```python
from build123d import *

# Parameters (mm, degrees)
SKETCH1_W               = 12.409227922
SKETCH1_H               = 27.718567262
SKETCH1_R               = 1
SKETCH1_W_2             = 8
SKETCH1_H_2             = 18.5
BOSS_EXTRUDE1_DEPTH     = 10
SKETCH6_W               = 12.409227922
SKETCH6_H               = 4.603346058
BOSS_EXTRUDE3_DEPTH     = 15
SKETCH7_R               = 3.1
CUT_EXTRUDE4_DEPTH      = 2.25
SKETCH8_W               = 11.323212184
SKETCH8_H               = 4
CUT_EXTRUDE5_DEPTH      = 1.25
CUT_EXTRUDE7_DEPTH      = 31.392767012
CUT_EXTRUDE7_DEPTH_BACK = 31.392767012
SKETCH9_R               = 1.5
SKETCH9_R_2             = 0.5
FILLET2_R               = 5
SKETCH10_R              = 3.380365375
CUT_EXTRUDE8_DEPTH      = 0.5
CHAMFER3_SIZE           = 2
FILLET3_R               = 5


with BuildPart() as part:
    # Sketch1 → Boss-Extrude1 (new body)
    with BuildSketch(Plane(origin=(0, 0, 0), x_dir=(0, 0, -1), z_dir=(1, 0, 0))):
        with Locations((1.233520205, 9.89974551)):
            Rectangle(SKETCH1_W, SKETCH1_H)
        with Locations((1.233520205, 20.798227972)):
            Circle(SKETCH1_R, mode=Mode.SUBTRACT)
        with Locations((1.233520205, -1.111772028)):
            Circle(SKETCH1_R, mode=Mode.SUBTRACT)
        with Locations((1.233520205, 9.843227972)):
            Rectangle(SKETCH1_W_2, SKETCH1_H_2, mode=Mode.SUBTRACT)
    extrude(amount=BOSS_EXTRUDE1_DEPTH)

    # Sketch6 → Boss-Extrude3 (add)
    with BuildSketch(Plane.ZY):
        with Locations((-1.233520205, 21.457356112)):
            Rectangle(SKETCH6_W, SKETCH6_H)
    extrude(amount=BOSS_EXTRUDE3_DEPTH)

    # Sketch7 → Cut-Extrude4 (cut)
    with BuildSketch(Plane.XZ.offset(-19.155683083)):
        with Locations(Location((-9.660045294, -1.233520205, 0), (0, 0, 270))):
            Circle(SKETCH7_R)
    extrude(amount=-CUT_EXTRUDE4_DEPTH, mode=Mode.SUBTRACT)

    # Sketch8 → Cut-Extrude5 (cut)
    with BuildSketch(Plane.XZ.offset(-19.155683083)):
        with Locations((-5.661606092, -1.303442539)):
            Rectangle(SKETCH8_W, SKETCH8_H)
    extrude(amount=-CUT_EXTRUDE5_DEPTH, mode=Mode.SUBTRACT)

    # Sketch9 → Cut-Extrude7 (cut, two sides: drawn at the far end of the back side and taken through both)
    with BuildSketch(Plane.XZ.offset(-21.405683083).offset(-CUT_EXTRUDE7_DEPTH_BACK)):
        with Locations(Location((-9.660045294, -1.233520205, 0), (0, 0, 270))):
            Circle(SKETCH9_R)
        with Locations(Location((-1.660045294, -1.233520205, 0), (0, 0, 270))):
            Circle(SKETCH9_R_2)
    extrude(amount=CUT_EXTRUDE7_DEPTH + CUT_EXTRUDE7_DEPTH_BACK, mode=Mode.SUBTRACT)

    # Fillet2
    fillet2_edges = [part.edges().sort_by_distance(p)[0] for p in [
        (-15, 21.457356112, -7.438134166),
        (-15, 21.457356112, 4.971093756),
    ]]
    fillet(fillet2_edges, radius=FILLET2_R)

    # Sketch10 → Cut-Extrude8 (cut)
    with BuildSketch(Plane(origin=(0, 23.759029141, 0), x_dir=(1, 0, 0), z_dir=(0, 1, 0))):
        with Locations(Location((-9.660045294, 1.233520205, 0), (0, 0, 270))):
            Circle(SKETCH10_R)
    extrude(amount=-CUT_EXTRUDE8_DEPTH, mode=Mode.SUBTRACT)

    # Chamfer3
    # the kernel refuses this chamfer: 2 mm, written as the material it takes off along each edge
    with BuildSketch(Plane(origin=(-5.143365976, -3.959538121, -7.438134166), x_dir=(0, 0.9996219169112968, -0.027495876610586487), z_dir=(1, 0, 0))) as chamfer3_piece_1:
        Polygon((CHAMFER3_SIZE * 0.999621916911, CHAMFER3_SIZE * 0.0274958766106), (-CHAMFER3_SIZE * 0.0274958766106, CHAMFER3_SIZE * 0.999621916911), (0, 0), align=None)
    extrude(amount=20.286731952, mode=Mode.SUBTRACT)
    with BuildSketch(Plane(origin=(-5.143365976, -3.959538121, 4.971093756), x_dir=(0, 0.9996219169112968, 0.027495876610586487), z_dir=(1, 0, 0))) as chamfer3_piece_2:
        Polygon((CHAMFER3_SIZE * 0.999621916911, -CHAMFER3_SIZE * 0.0274958766106), (-CHAMFER3_SIZE * 0.0274958766106, -CHAMFER3_SIZE * 0.999621916911), (0, 0), align=None)
    extrude(amount=20.286731952, mode=Mode.SUBTRACT)
    with BuildSketch(Plane(origin=(-10, 23.759029141, 4.971093756), x_dir=(0, 0.02749587661058563, -0.9996219169112968), z_dir=(1, 0, 0)), Plane(origin=(15.143365976, 23.759029141, -7.438134166), x_dir=(0, 0.027495876610585623, 0.9996219169112968), z_dir=(-1, 0, 0))) as chamfer3_piece_3:
        Polygon((CHAMFER3_SIZE * 0.999621916911, -CHAMFER3_SIZE * 0.0274958766106), (-CHAMFER3_SIZE * 0.0274958766106, -CHAMFER3_SIZE * 0.999621916911), (0, 0), align=None)
    extrude(amount=25.143365976, mode=Mode.SUBTRACT)
    with BuildSketch(Plane(origin=(-15, 23.759029141, -2.438134166), x_dir=(0.9996219169112968, 0.027495876610585623, 0), z_dir=(0, 0, 1))) as chamfer3_piece_4:
        Polygon((CHAMFER3_SIZE * 0.999621916911, -CHAMFER3_SIZE * 0.0274958766106), (-CHAMFER3_SIZE * 0.0274958766106, -CHAMFER3_SIZE * 0.999621916911), (0, 0), align=None)
    extrude(amount=2.409227923, mode=Mode.SUBTRACT)
    with BuildSketch(Plane(origin=(-10, 23.759029141, -0.028906244), x_dir=(-1, 0, 0), z_dir=(0, 0, -1))) as chamfer3_piece_5:
        Polygon((5 - CHAMFER3_SIZE, 0), (5, -CHAMFER3_SIZE), (5, 0), align=None)
    revolve(axis=Axis((-10, 23.759029141, -0.028906244), (0, 1, 0)), revolution_arc=90, mode=Mode.SUBTRACT)
    with BuildSketch(Plane(origin=(-10, 23.759029141, -2.438134166), x_dir=(-1, 0, 0), z_dir=(0, 0, 1))) as chamfer3_piece_6:
        Polygon((5 - CHAMFER3_SIZE, 0), (5, CHAMFER3_SIZE), (5, 0), align=None)
    revolve(axis=Axis((-10, 23.759029141, -2.438134166), (0, -1, 0)), revolution_arc=90, mode=Mode.SUBTRACT)

    # Fillet3
    # the kernel refuses this fillet: 5 mm, written as the material it adds along each edge
    with BuildSketch(Plane(origin=(0, 19.155683083, 9.196557461), x_dir=(-1, 0, 0), z_dir=(0, 0, -1))) as fillet3_piece_1_section:
        with BuildLine():
            CenterArc((FILLET3_R, -FILLET3_R), FILLET3_R, 90, 90)
            Line((0, -FILLET3_R), (0, 0))
            Line((0, 0), (FILLET3_R, 0))
        make_face()
    fillet3_piece_1 = extrude(amount=29.134691627, mode=Mode.PRIVATE)
    fillet3_piece_1 = split(fillet3_piece_1, bisect_by=Plane(origin=(-2.240914142, 19.125188019, 4.971093756), z_dir=(0, 0, -1)), keep=Keep.TOP, mode=Mode.PRIVATE)
    fillet3_piece_1 = split(fillet3_piece_1, bisect_by=Plane(origin=(-2.240914142, 19.093227972, 3.868786776), z_dir=(0, 1, 0)), keep=Keep.TOP, mode=Mode.PRIVATE)
    fillet3_piece_1 = split(fillet3_piece_1, bisect_by=Plane(origin=(-2.240914142, 19.125188019, 0.696557461), z_dir=(0, 0, 1)), keep=Keep.TOP, mode=Mode.PRIVATE)
    add(fillet3_piece_1)
    with BuildSketch(Plane(origin=(0, 19.155683083, 9.196557461), x_dir=(-1, 0, 0), z_dir=(0, 0, -1))) as fillet3_piece_2_section:
        with BuildLine():
            CenterArc((FILLET3_R, -FILLET3_R), FILLET3_R, 90, 90)
            Line((0, -FILLET3_R), (0, 0))
            Line((0, 0), (FILLET3_R, 0))
        make_face()
    fillet3_piece_2 = extrude(amount=29.134691627, mode=Mode.PRIVATE)
    fillet3_piece_2 = split(fillet3_piece_2, bisect_by=Plane(origin=(-1.055076688, 17.979153471, 4.971093756), z_dir=(0, 0, -1)), keep=Keep.TOP, mode=Mode.PRIVATE)
    fillet3_piece_2 = split(fillet3_piece_2, bisect_by=Plane(origin=(-1.055076688, 17.979153471, 2.766479795), z_dir=(0, 0, 1)), keep=Keep.TOP, mode=Mode.PRIVATE)
    add(fillet3_piece_2)
    with BuildSketch(Plane(origin=(0, 19.155683083, -3.303442539), x_dir=(-1, 0, 0), z_dir=(0, 0, -1))) as fillet3_piece_3_section:
        with BuildLine():
            CenterArc((FILLET3_R, -FILLET3_R), FILLET3_R, 90, 90)
            Line((0, -FILLET3_R), (0, 0))
            Line((0, 0), (FILLET3_R, 0))
        make_face()
    fillet3_piece_3 = extrude(amount=4.134691627, mode=Mode.PRIVATE)
    fillet3_piece_3 = split(fillet3_piece_3, bisect_by=Plane(origin=(-2.240914142, 19.093227972, -4.268481372), z_dir=(0, 1, 0)), keep=Keep.TOP, mode=Mode.PRIVATE)
    add(fillet3_piece_3)
    with BuildSketch(Plane(origin=(0, 19.155683083, 9.196557461), x_dir=(-1, 0, 0), z_dir=(0, 0, -1))) as fillet3_piece_4_section:
        with BuildLine():
            CenterArc((FILLET3_R, -FILLET3_R), FILLET3_R, 90, 90)
            Line((0, -FILLET3_R), (0, 0))
            Line((0, 0), (FILLET3_R, 0))
        make_face()
    fillet3_piece_4 = extrude(amount=16.634691627, mode=Mode.PRIVATE)
    fillet3_piece_4 = split(fillet3_piece_4, bisect_by=Plane(origin=(-1.055076688, 17.979153471, -5.233520205), z_dir=(0, 0, -1)), keep=Keep.TOP, mode=Mode.PRIVATE)
    add(fillet3_piece_4)
    with BuildSketch(Plane(origin=(0, 19.155683083, 4.971093756), x_dir=(-1, 0, 0), z_dir=(0, 0, -1))) as fillet3_piece_5_section:
        with BuildLine():
            CenterArc((FILLET3_R, -FILLET3_R), FILLET3_R, 90, 90)
            Line((0, -FILLET3_R), (0, 0))
            Line((0, 0), (FILLET3_R, 0))
        make_face()
    fillet3_piece_5 = extrude(amount=4.274536296, mode=Mode.PRIVATE)
    fillet3_piece_5 = split(fillet3_piece_5, bisect_by=Plane(origin=(-2.240914142, 19.093227972, 3.868786776), z_dir=(0, 1, 0)), keep=Keep.TOP, mode=Mode.PRIVATE)
    add(fillet3_piece_5)
    with BuildSketch(Plane(origin=(0, 19.155683083, 4.971093756), x_dir=(-1, 0, 0), z_dir=(0, 0, -1))) as fillet3_piece_6_section:
        with BuildLine():
            CenterArc((FILLET3_R, -FILLET3_R), FILLET3_R, 90, 90)
            Line((0, -FILLET3_R), (0, 0))
            Line((0, 0), (FILLET3_R, 0))
        make_face()
    fillet3_piece_6 = extrude(amount=16.774536296, mode=Mode.PRIVATE)
    fillet3_piece_6 = split(fillet3_piece_6, bisect_by=Plane(origin=(-1.055076688, 17.979153471, 2.766479795), z_dir=(0, 0, 1)), keep=Keep.TOP, mode=Mode.PRIVATE)
    add(fillet3_piece_6)
    with BuildSketch(Plane(origin=(0, 19.155683083, 17.471093756), x_dir=(-1, 0, 0), z_dir=(0, 0, -1))) as fillet3_piece_7_section:
        with BuildLine():
            CenterArc((FILLET3_R, -FILLET3_R), FILLET3_R, 90, 90)
            Line((0, -FILLET3_R), (0, 0))
            Line((0, 0), (FILLET3_R, 0))
        make_face()
    fillet3_piece_7 = extrude(amount=29.274536296, mode=Mode.PRIVATE)
    fillet3_piece_7 = split(fillet3_piece_7, bisect_by=Plane(origin=(-2.240914142, 19.125188019, -7.438134166), z_dir=(0, 0, 1)), keep=Keep.TOP, mode=Mode.PRIVATE)
    fillet3_piece_7 = split(fillet3_piece_7, bisect_by=Plane(origin=(-2.240914142, 19.093227972, -4.268481372), z_dir=(0, 1, 0)), keep=Keep.TOP, mode=Mode.PRIVATE)
    fillet3_piece_7 = split(fillet3_piece_7, bisect_by=Plane(origin=(-2.240914142, 19.125188019, -3.303442539), z_dir=(0, 0, -1)), keep=Keep.TOP, mode=Mode.PRIVATE)
    add(fillet3_piece_7)
    with BuildSketch(Plane(origin=(0, 19.155683083, 17.471093756), x_dir=(-1, 0, 0), z_dir=(0, 0, -1))) as fillet3_piece_8_section:
        with BuildLine():
            CenterArc((FILLET3_R, -FILLET3_R), FILLET3_R, 90, 90)
            Line((0, -FILLET3_R), (0, 0))
            Line((0, 0), (FILLET3_R, 0))
        make_face()
    fillet3_piece_8 = extrude(amount=29.274536296, mode=Mode.PRIVATE)
    fillet3_piece_8 = split(fillet3_piece_8, bisect_by=Plane(origin=(-1.055076688, 17.979153471, -7.438134166), z_dir=(0, 0, 1)), keep=Keep.TOP, mode=Mode.PRIVATE)
    fillet3_piece_8 = split(fillet3_piece_8, bisect_by=Plane(origin=(-1.055076688, 17.979153471, -5.233520205), z_dir=(0, 0, -1)), keep=Keep.TOP, mode=Mode.PRIVATE)
    add(fillet3_piece_8)


solid = part.part
```
Input: part model. Units: mm. Frame: model coordinates. A direction names the side the tool comes from. Round coordinates to 2 decimals unless told otherwise and drop trailing zeros. Write each loop counter-clockwise with the first axis right and the second up, starting at its lowest first coordinate (ties: lowest second). Pieces come first, ordered by that corner, then holes. Notation, with made-up numbers: (2.5, 79.25) - (7.5, 79.25) arc R25 ccw to (7.5, 106.25) - close; hole circle Ø7 at (80, 46). An arc over 180 degrees is marked (long way). Write item = value, one per line.
(1) Material intervals for probe 1 along Y at (x, z) = (7.75, 2.25); probe 2 along Z at (x, y) = (5, 9.25); probe 3 along X at (y, z) = (19.5, -1), sorted ascending.
Geometry check:
probe_1 = -3.96 to 0.59, 19.09 to 23.76
probe_2 = -7.44 to -5.23, 2.77 to 4.97
probe_3 = -15 to -12.75, 0 to 10
(2) Access query for faces 1 (the flat face through (0, 21, -1)), 2 (the flat face through (-9, 21.406, -3)), 3 (the flat face through (4, 13, -7.438)), 4 (the flat face through (5, 10, -5.234)). Directions: +Z, -Z, +X, -X, +Y, -Y. A direction counts if a zero-diameter tool reaches every point of the face in a straight line with its end or side. Return the directions, or none.
Geometry check:
face_1 = +X
face_2 = -Y
face_3 = -Z, +X, -X, +Y, -Y
face_4 = +X, -X
(3) Contact query for flat-ended pins moving along their axis: pin 1 Ø5 at (x, z) = (-9.66, -1.23) entering from +Y; pin 2 Ø3 at (x, z) = (-8.5, 0.5) entering from -Y; pin 3 Ø3 at (x, z) = (-2.5, -1.5) entering from -Y. Output: stop coordinate, or through.
Geometry check:
pin_1 = 23.26
pin_2 = 19.16
pin_3 = 20.41
(4) Section query B-B on x = 7. Output: boundary loops of the cut face in (y, z), then the cut area to 3 significant figures.
Geometry check:
outline = (-3.96, -5.44) - (-1.96, -7.44) - (21.76, -7.44) - (23.76, -5.44) - (23.76, 2.97) - (21.76, 4.97) - (-1.96, 4.97) - (-3.96, 2.97) - close; hole circle Ø2 at (-1.11, -1.23); hole (0.59, -5.23) - (19.09, -5.23) - (19.09, 2.77) - (0.59, 2.77) - close; hole circle Ø2 at (20.8, -1.23)
area = 182 mm^2
(5) Pull-direction query (X, two-part tool) for faces 5 (the flat face through (-4, 20.406, -1)), 6 (the cylindrical face through (4.93, 21.79, -1.1)), 7 (the flat face through (0, 3, 3)); classes: +X half, -X half, draft (parallel to the pull), parting line (faces both ways), or undercut.
Geometry check:
face_5 = undercut
face_6 = draft
face_7 = -X half
(6) Section query A-A on y = 5. Output: boundary loops of the cut face in (x, z).
Geometry check:
outline = (0, -7.44) - (10, -7.44) - (10, -5.23) - (0, -5.23) - close; (0, 2.77) - (10, 2.77) - (10, 4.97) - (0, 4.97) - close
